Read the model definition and answer for the solid it produces. Units are mm, in the model's axes. Give positions to 0.01 mm unless a question says otherwise; leave off trailing zeros. Write each loop counter-clockwise with the first axis right and the second up, starting at its lowest first coordinate (ties: lowest second). Pieces come first, ordered by that corner, then holes.
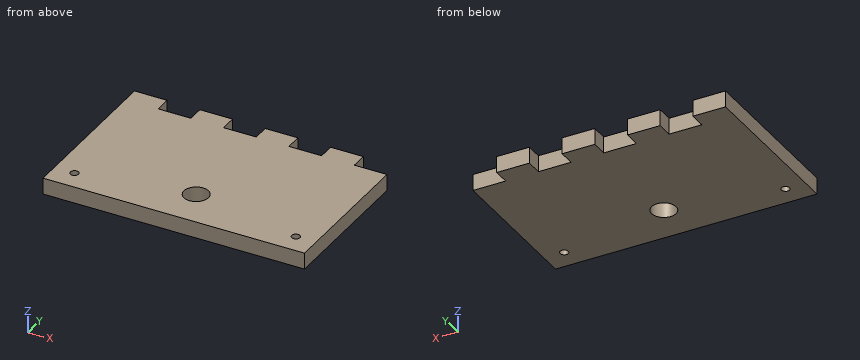
Autodesk Inventor part; units mm, degrees
ref_plane "YZ Plane" through (0, 0, 0) normal (1, 0, 0) x (0, 1, 0)
ref_plane "XZ Plane" through (0, 0, 0) normal (0, 1, 0) x (-1, 0, 0)
ref_plane "XY Plane" through (0, 0, 0) normal (0, 0, 1) x (1, 0, 0)
sketch "Sketch1" plane through (0, 0, 0) normal (0, 0, 1) x (1, 0, 0)
  circle A0 centre (0, 7.8) radius 4.7625
  circle A1 centre (-43, 0) radius 1.5875
  circle A2 centre (43, 0) radius 1.5875
  line L0 (-50.8, 56.695) -> (-38.1, 56.695)
  line L1 (50.8, -8.075) -> (-50.8, -8.075)
  line L2 (-50.8, -8.075) -> (-50.8, 56.695)
  line L3 (-50.8, 56.695) -> (-38.1, 56.695)
  line L4 (-38.1, 56.695) -> (-38.1, 50.345)
  line L5 (-50.8, 50.345) -> (-50.8, 56.695)
  line L6 (-38.1, 50.345) -> (-25.4, 50.345)
  line L7 (-25.4, 50.345) -> (-25.4, 56.695)
  line L8 (-38.1, 56.695) -> (-38.1, 50.345)
  line L9 (-12.7, 50.345) -> (-12.7, 56.695)
  line L10 (-12.7, 56.695) -> (-25.4, 56.695)
  line L11 (-25.4, 56.695) -> (-25.4, 50.345)
  line L12 (0, 56.695) -> (0, 50.345)
  line L13 (0, 50.345) -> (-12.7, 50.345)
  line L14 (-12.7, 50.345) -> (-12.7, 56.695)
  line L15 (12.7, 50.345) -> (12.7, 56.695)
  line L16 (12.7, 56.695) -> (0, 56.695)
  line L17 (0, 56.695) -> (0, 50.345)
  line L18 (25.4, 56.695) -> (25.4, 50.345)
  line L19 (25.4, 50.345) -> (12.7, 50.345)
  line L20 (12.7, 50.345) -> (12.7, 56.695)
  line L21 (25.4, 56.695) -> (38.1, 56.695)
  line L22 (38.1, 56.695) -> (38.1, 50.345)
  line L23 (25.4, 50.345) -> (25.4, 56.695)
  line L24 (38.1, 50.345) -> (50.8, 50.345)
  line L25 (38.1, 56.695) -> (38.1, 50.345)
  line L26 (0, 56.695) -> (12.7, 56.695)
  line L27 (25.4, 56.695) -> (38.1, 56.695)
  line L28 (50.8, 50.345) -> (50.8, -8.075)
  point P0 (0, 0)
  dimension "d0" = 9.525
  dimension "d1" = 3.175
  dimension "d2" = 3.175
  dimension "d6" = 0
  dimension "d7" = 101.6
  dimension "d13" = 43
  dimension "d14" = 43
  dimension "d16" = 15.875
  dimension "d17" = 7.8
  dimension "d18" = 7.8
  dimension "d19" = 48.895
  dimension "d21" = 12.7
  dimension "d22" = 6.35
  dimension "d23" = 12.7
  dimension "d24" = 12.7
  dimension "d25" = 6.35
  dimension "d26" = 6.35
  dimension "d27" = 12.7
  dimension "d28" = 6.35
  dimension "d29" = 12.7
  dimension "d30" = 6.35
  dimension "d31" = 12.7
  dimension "d32" = 6.35
extrude "Extrusion1" add sketch "Sketch1" along normal blind 6.35
sketch "Sketch2" plane through (-50.8, 56.695, 0) normal (0, 1, 0) x (1, 0, 0)
  point P0 (50.8, 0)
properties part number "structural" material "Polycarbonate, Clear"
Item 1: Section B-B (y = 0) is taken. Write down the section's boundary in (x, z).
Result set:
outline: (-50.8, 0) - (-44.59, 0) - (-44.59, 6.35) - (-50.8, 6.35) - close; (-41.41, 0) - (41.41, 0) - (41.41, 6.35) - (-41.41, 6.35) - close; (44.59, 0) - (50.8, 0) - (50.8, 6.35) - (44.59, 6.35) - close
Item 2: Find the intervals of material crossed by line 1 along Y through (x, z) = (43, 3) (1 decimal); line 2 along Y through (x, z) = (-5, 2) (3 decimals); line 3 along X through (y, z) = (9.5, 4.75), in increasing order.
Result set:
line 1: y = -8.1 to -1.6, 1.6 to 50.3
line 2: y = -8.075 to 50.345
line 3: x = -50.8 to -4.45, 4.45 to 50.8
Item 3: Section D-D (y = 7.8) is taken. Write down the section's boundary in (x, z), and give its area (3 significant figures).
Result set:
outline: (-50.8, 0) - (-4.76, 0) - (-4.76, 6.35) - (-50.8, 6.35) - close; (4.76, 0) - (50.8, 0) - (50.8, 6.35) - (4.76, 6.35) - close
area: 585 mm2
Item 4: Section C-C (z = 1.5) is taken. Write down the section's boundary in (x, y) (1 decimal).
Result set:
outline: (-50.8, -8.1) - (50.8, -8.1) - (50.8, 50.3) - (38.1, 50.3) - (38.1, 56.7) - (25.4, 56.7) - (25.4, 50.3) - (12.7, 50.3) - (12.7, 56.7) - (0, 56.7) - (0, 50.3) - (-12.7, 50.3) - (-12.7, 56.7) - (-25.4, 56.7) - (-25.4, 50.3) - (-38.1, 50.3) - (-38.1, 56.7) - (-50.8, 56.7) - close; hole circle Ø3.2 at (-43, 0); hole circle Ø9.5 at (0, 7.8); hole circle Ø3.2 at (43, 0)
Item 5: Each of these flat-tipped pins is pushed along its axis until it touches: pin 1 Ø12 at (x, y) = (-35.5, 5) entering from -Z; pin 2 Ø1.9 at (x, z) = (21, 4) entering from +Y (3 decimals); pin 3 Ø3 at (y, z) = (54.5, 4) entering from +X. Where does it stop, or does it pass through?
Result set:
pin 1: stops at z = 0
pin 2: stops at y = 50.345
pin 3: stops at x = 38.1
